Answer from the drawing. Dimensions are ordinates in mm from the lowest x, y and z of the part. A direction names the side the tool comes from. Coordinates: 2 decimals unless noted, no trailing zeros. Order: outer loops, then holes, each group sorted by start corner. A loop starts at its lowest first (then second) coordinate and runs counter-clockwise, first axis right, second up. Notation, with made-up numbers: (-6, -26.75) -> (51, -26.75) arc R11 cw to (51, -22.75) -> close; hole circle Ø4 at (5.25, -37.75). An arc over 180 degrees is marked (long way). Answer in a Markdown table with one row per item.
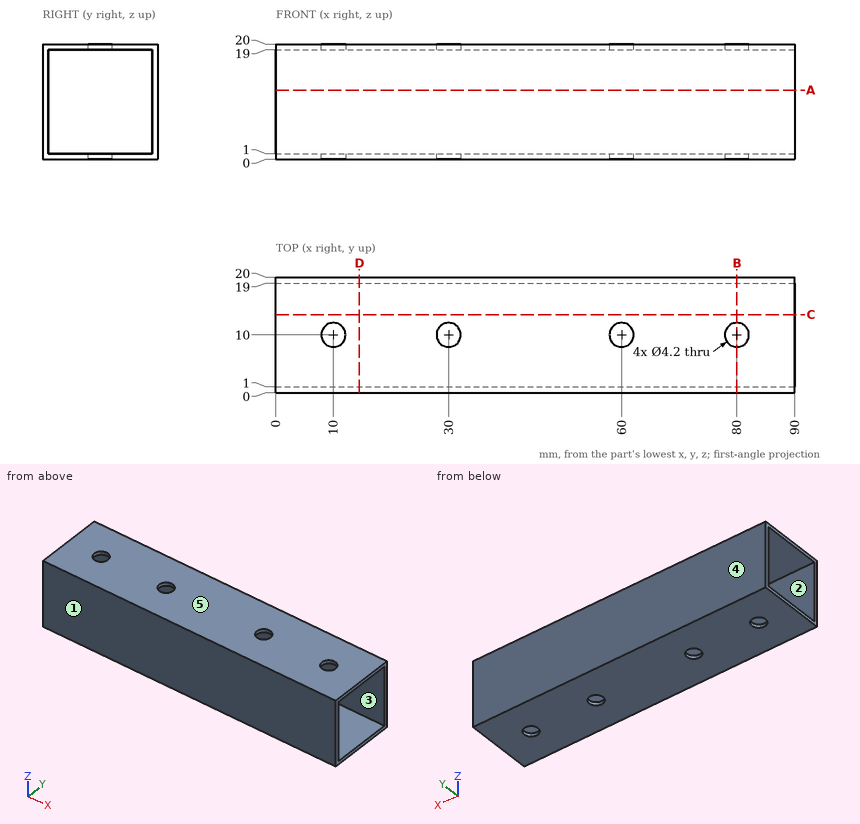
Q1. The part is cut by section B-B (x = 80). Write down the section's boundary in (y, z), then the cut area to 3 significant figures.
Outcome:
| item | result |
|---|---|
| outline | (0, 0) -> (7.9, 0) -> (7.9, 1) -> (1, 1) -> (1, 19) -> (7.9, 19) -> (7.9, 20) -> (0, 20) -> close; (12.1, 0) -> (20, 0) -> (20, 20) -> (12.1, 20) -> (12.1, 19) -> (19, 19) -> (19, 1) -> (12.1, 1) -> close |
| area | 67.6 mm² |
Q2. The part is cut by section D-D (x = 14.5). Write down the section's boundary in (y, z).
Outcome:
| item | result |
|---|---|
| outline | (0, 0) -> (20, 0) -> (20, 20) -> (0, 20) -> close; hole (1, 1) -> (19, 1) -> (19, 19) -> (1, 19) -> close |
Q3. Consider line 1 (Y direction, x = 49, z = 16.5); line 2 (Y direction, x = 10, z = 0.6). Determine where each line is inside the solid, lowest interval first.
Outcome:
| item | result |
|---|---|
| line 1 | 0 to 1, 19 to 20 |
| line 2 | 0 to 7.9, 12.1 to 20 |
Q4. For a pull along Z with two mould halves and no side action, classify the marked faces 3, 4 and 5 as pulls with the +Z half, pulls with the -Z half, needs draft (parallel to the pull), parting line crosses it, or undercut.
Outcome:
| item | result |
|---|---|
| face 3 | undercut |
| face 4 | needs draft |
| face 5 | pulls with the +Z half |
Q5. Given pin 1 (2.5 mm diameter, centred on x = 80, y = 10, fed in from -Z), flat-ended and moving along its own axis, determine where the tip first touches the part or whether it passes through.
Outcome:
| item | result |
|---|---|
| pin 1 | through |
Q6. The part is cut by section A-A (z = 12). Write down the section's boundary in (x, y).
Outcome:
| item | result |
|---|---|
| outline | (0, 0) -> (90, 0) -> (90, 1) -> (0, 1) -> close; (0, 19) -> (90, 19) -> (90, 20) -> (0, 20) -> close |
Q7. For the marked faces 1 and 2, determine the directions among +Z, -Z, +X, -X, +Y, -Y from which every point of the face is accessible in a straight line to the end or side of a thin tool.
Outcome:
| item | result |
|---|---|
| face 1 | +Z, -Z, +X, -X, -Y |
| face 2 | +X, -X |
